The model under review builds one solid part; all positions refer to its coordinate system, in mm. Give positions to 0.01 mm unless a question says otherwise; leave off trailing zeros. Write each loop counter-clockwise with the first axis right and the second up, starting at its lowest first coordinate (ties: lowest second). Pieces come first, ordered by that corner, then holes.
from build123d import *

# Parameters (mm, degrees)
SKETCH1_W          = 190.3
SKETCH1_H          = 121.4
SKETCH1_W_2        = 166.3
SKETCH1_H_2        = 101.4
EXTRUDE1_DEPTH     = 3
FILLET1_R          = 5
SKETCH2_R          = 1.75
CUT_EXTRUDE1_DEPTH = 3


with BuildPart() as part:
    # Sketch1 → Extrude1 (new body)
    with BuildSketch(Plane(origin=(0, 0, 0), x_dir=(1, 0, 0), z_dir=(0, 1, 0))):
        Rectangle(SKETCH1_W, SKETCH1_H)
        Rectangle(SKETCH1_W_2, SKETCH1_H_2, mode=Mode.SUBTRACT)
    extrude(amount=EXTRUDE1_DEPTH)

    # Fillet1
    fillet1_edges = [part.edges().sort_by_distance(p)[0] for p in [
        (-95.15, 1.5, -60.7),
        (95.15, 1.5, -60.7),
        (95.15, 1.5, 60.7),
        (-95.15, 1.5, 60.7),
    ]]
    fillet(fillet1_edges, radius=FILLET1_R)

    # Sketch2 → Cut-Extrude1 (cut)
    with BuildSketch(Plane(origin=(-128.478742323, 3, 300.3), x_dir=(1, 0, 0), z_dir=(0, 1, 0))):
        with Locations(Location((38.428742323, 339.6, 0), (0, 0, 270))):
            Circle(SKETCH2_R)
        with Locations(Location((218.528742323, 339.6, 0), (0, 0, 270))):
            Circle(SKETCH2_R)
        with Locations(Location((218.528742323, 261, 0), (0, 0, 270))):
            Circle(SKETCH2_R)
        with Locations(Location((38.428742323, 261, 0), (0, 0, 270))):
            Circle(SKETCH2_R)
    extrude(amount=-CUT_EXTRUDE1_DEPTH, mode=Mode.SUBTRACT)


solid = part.part
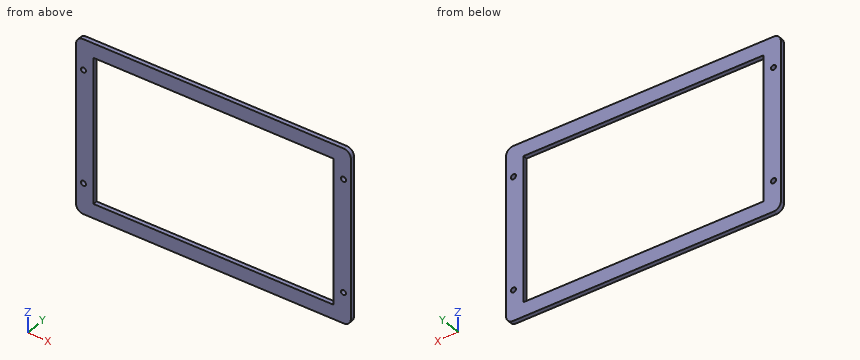
1) Consider section C-C, the plane y = 1.1. Give the boundary of the cut face in (x, z), then the cut area to 3 significant figures.
2) Consider section A-A, the plane x = 11.5. Give the boundary of the cut face in (y, z), then the cut area to 3 significant figures.
3) To check wall thickness, follow probe 1 along Z at (x, y) = (90.05, 0.7); probe 2 along X at (y, z) = (1.85, -39.3); probe 3 along X at (y, z) = (1.6, -7). State the ranges of each line that lie inside material, in increasing order.
4) Consider section B-B, the plane z = 28. Give the boundary of the cut face in (x, y), then the cut area to 3 significant figures.
Answer block:
1. outline: (-95.15, -55.7) arc R5 ccw to (-90.15, -60.7) - (90.15, -60.7) arc R5 ccw to (95.15, -55.7) - (95.15, 55.7) arc R5 ccw to (90.15, 60.7) - (-90.15, 60.7) arc R5 ccw to (-95.15, 55.7) - close; hole circle Ø3.5 at (-90.05, -39.3); hole circle Ø3.5 at (-90.05, 39.3); hole (-83.15, -50.7) - (83.15, -50.7) - (83.15, 50.7) - (-83.15, 50.7) - close; hole circle Ø3.5 at (90.05, -39.3); hole circle Ø3.5 at (90.05, 39.3)
1. area: 6,180 mm2
2. outline: (0, -60.7) - (3, -60.7) - (3, -50.7) - (0, -50.7) - close; (0, 50.7) - (3, 50.7) - (3, 60.7) - (0, 60.7) - close
2. area: 60.0 mm2
3. probe 1: z = -60.7 to -41.05, -37.55 to 37.55, 41.05 to 60.7
3. probe 2: x = -95.15 to -91.8, -88.3 to -83.15, 83.15 to 88.3, 91.8 to 95.15
3. probe 3: x = -95.15 to -83.15, 83.15 to 95.15
4. outline: (-95.15, 0) - (-83.15, 0) - (-83.15, 3) - (-95.15, 3) - close; (83.15, 0) - (95.15, 0) - (95.15, 3) - (83.15, 3) - close
4. area: 72.0 mm2
